Geometry: final body of the model. Coordinates: model frame, mm. A direction names the side the tool comes from. Coordinates: 2 decimals unless noted, no trailing zeros. Order: outer loops, then holes, each group sorted by start corner. A loop starts at its lowest first (then second) coordinate and runs counter-clockwise, first axis right, second up. Notation, with made-up numbers: (-24.5, -21) - (-15.5, -21) arc R15 cw to (-15.5, -8) - close; hole circle Ø6 at (15.25, -28.75). An arc over 180 degrees is marked (long way). Use a Markdown table: item, result. Add a question column.
Autodesk Inventor part; units mm, degrees
ref_plane "YZ Plane" through (0, 0, 0) normal (1, 0, 0) x (0, 1, 0)
ref_plane "XZ Plane" through (0, 0, 0) normal (0, 1, 0) x (-1, 0, 0)
ref_plane "XY Plane" through (0, 0, 0) normal (0, 0, 1) x (1, 0, 0)
sketch "Sketch1" plane through (0, 0, 0) normal (0, 0, 1) x (1, 0, 0)
  line L0 (0, 0) -> (150, 0)
  line L1 (150, 0) -> (150, 30)
  line L2 (150, 30) -> (25, 30)
  line L3 (25, 30) -> (25, 70)
  line L4 (25, 70) -> (0, 70)
  line L5 (0, 70) -> (0, 0)
  dimension "d0" = 150
  dimension "d1" = 30
  dimension "d2" = 125
  dimension "d3" = 40
extrude "Extrusion1" add sketch "Sketch1" along normal blind 60
sketch "Sketch2" plane through (150, 0, 0) normal (1, 0, 0) x (0, 0, -1)
  line L0 (0, 30) -> (-60, 30)
  line L1 (-40, 30) -> (-20, 30)
  line L2 (-20, 30) -> (-20, 20)
  line L3 (-20, 20) -> (-40, 20)
  line L4 (-40, 20) -> (-40, 30)
  point P0 (0, 0)
  dimension "d6" = 20
  dimension "d7" = 10
extrude "Extrusion2" cut sketch "Sketch2" against normal blind 125
sketch "Sketch3" plane through (0, 0, 0) normal (0, -1, 0) x (1, 0, 0)
  circle A0 centre (75, 30) radius 6
  point P0 (0, 0)
  dimension "d10" = 12
extrude "Extrusion3" cut sketch "Sketch3" against normal blind 15
sketch "Sketch4" plane through (25, 30, 0) normal (1, 0, 0) x (0, 0, -1)
  circle A0 centre (-30, 20) radius 3.25
  point P0 (0, -30)
  dimension "d13" = 6.5
extrude "Extrusion4" cut sketch "Sketch4" against normal blind 47.5
properties part number "sabit_govde"
1) Section C-C (x = 29). Return loops of the section in (y, z).
2) Ray query, line 1 along X through (y, z) = (36, 43); line 2 along Y through (x, z) = (6.75, 30); line 3 along Y through (x, z) = (128, 33). Return the intervals inside material, ascending.
3) Pin query (flat end, axial travel): pin 1 (6 mm diameter, centred on x = 97.5, z = 47.5, fed in from +Y); pin 2 (3 mm diameter, centred on x = 75, z = 49.5, fed in from -Y); pin 3 (3.5 mm diameter, centred on x = 74, z = 29.5, fed in from -Y); pin 4 (9.5 mm diameter, centred on x = 75, z = 30, fed in from +Y). Return the tip coordinate at first contact, or that it passes through.
4) Section A-A (z = 30). Return loops of the section in (x, y).
5) Section B-B (y = 50). Return loops of the section in (x, z), then the cut area to 3 significant figures.
6) Draft query along X for faces 1 (the face through (75, 15, 30)), 2 (the face through (88, 25, 20)), 3 (the face through (0, 35, 30)). Return one class per face: pulls with the +X half, pulls with the -X half, needs draft (parallel to the pull), parting line crosses it, or undercut.
7) Section D-D (z = 51). Return loops of the section in (x, y), then the cut area to 3 significant figures.
8) Set-up query: faces 4 (the face through (69, 7, 30)), 5 (the face through (88, 30, 50)), 6 (the face through (74, 0, 23)), 7 (the face through (88, 20, 30)). Return all of +Z, -Z, +X, -X, +Y, -Y with unobstructed straight access to the full face (end or side cutting, diameter ignored); none if empty.
Values follow:
| question | item | result |
|---|---|---|
| 1 | outline | (0, 0) - (30, 0) - (30, 20) - (20, 20) - (20, 40) - (30, 40) - (30, 60) - (0, 60) - close |
| 2 | line 1 | x = 0 to 25 |
| 2 | line 2 | y = 0 to 46.75, 53.25 to 70 |
| 2 | line 3 | y = 0 to 20 |
| 3 | pin 1 | stops at y = 30 |
| 3 | pin 2 | stops at y = 0 |
| 3 | pin 3 | stops at y = 15 |
| 3 | pin 4 | stops at y = 20 |
| 4 | outline | (0, 0) - (69, 0) - (69, 15) - (81, 15) - (81, 0) - (150, 0) - (150, 20) - (25, 20) - (25, 46.75) - (0, 46.75) - close; (0, 53.25) - (25, 53.25) - (25, 70) - (0, 70) - close |
| 5 | outline | (0, 0) - (25, 0) - (25, 26.75) - (0, 26.75) - close; (0, 33.25) - (25, 33.25) - (25, 60) - (0, 60) - close |
| 5 | area | 1,340 mm² |
| 6 | face 1 | undercut |
| 6 | face 2 | needs draft |
| 6 | face 3 | pulls with the -X half |
| 7 | outline | (0, 0) - (150, 0) - (150, 30) - (25, 30) - (25, 70) - (0, 70) - close |
| 7 | area | 5,500 mm² |
| 8 | face 4 | -Y |
| 8 | face 5 | +Z, -Z, +X, +Y |
| 8 | face 6 | +Z, -Z, +X, -X, -Y |
| 8 | face 7 | +X, +Y |
